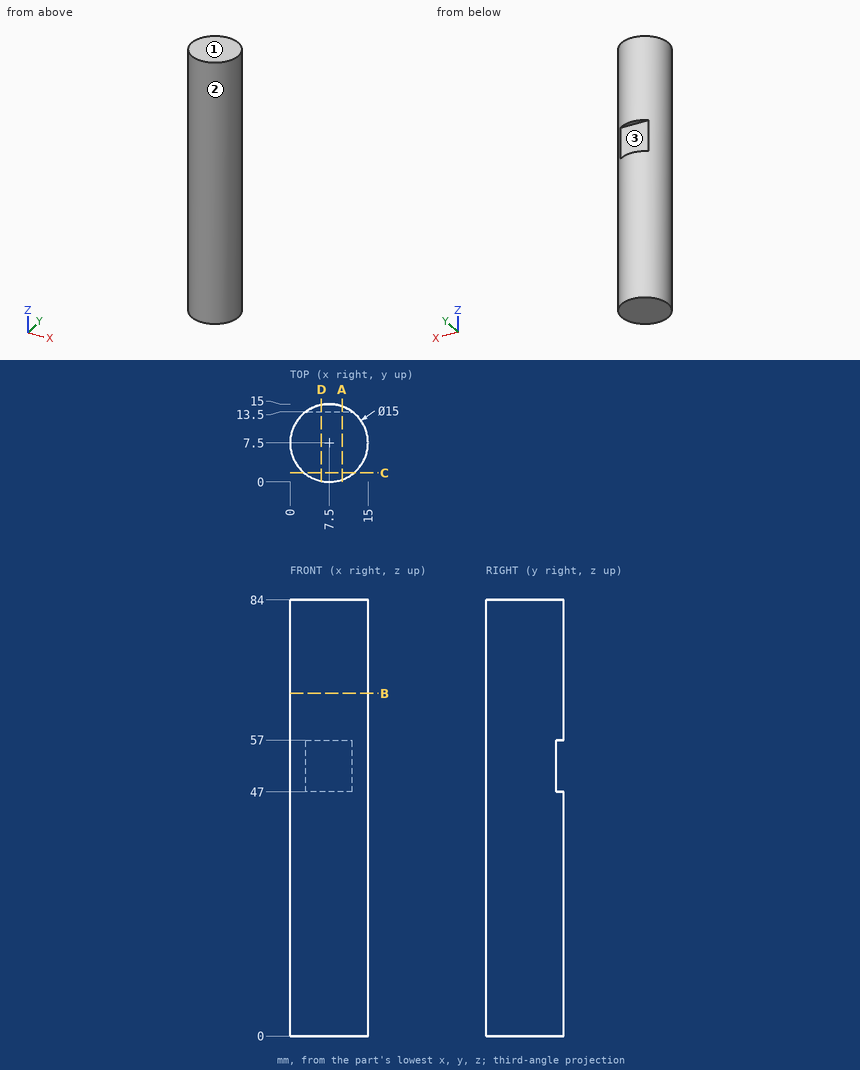
Print and shaded views of the part. All mm, measured from the part's lowest x, y and z. Give positions to 0.01 mm unless a question says otherwise; leave off trailing zeros. Loops run counter-clockwise (first coordinate to the right, second up) from the corner with the lowest first, then second, coordinate; pieces in that order, holes last.
1) Pull direction Z, two halves, no side cores. Call the marked faces 1, 2 and 3: +Z half, -Z half, draft (parallel to the pull), parting line (faces both ways), or undercut.
2) Wall check: line 1 (Z direction, x = 9, y = 13.75); line 2 (Y direction, x = 7, z = 50.5); line 3 (Y direction, x = 7, z = 35.5). Give the ranges that are in metal, low to high.
3) Flat gauge pins, fed straight in: pin 1 Ø3 at (x, z) = (4.5, 27) entering from +Y; pin 2 Ø2 at (y, z) = (10.5, 60.5) entering from -X; pin 3 Ø4.5 at (x, z) = (7.5, 52) entering from +Y. Where does each tip first touch, or does it go through?
4) Saw through at A-A (x = 10). Write the cut outline in (y, z), plus the area to 3 significant figures.
5) Saw through at C-C (y = 1.75). Write the cut outline in (x, z).
6) Saw through at B-B (z = 66). Write the cut outline in (x, y), plus the area to 3 significant figures.
7) Saw through at D-D (x = 6). Write the cut outline in (y, z), plus the area to 3 significant figures.
Answer block:
1. face 1: +Z half
1. face 2: draft
1. face 3: undercut
2. line 1: z = 0 to 47, 57 to 84
2. line 2: y = 0.02 to 13.5
2. line 3: y = 0.02 to 14.98
3. pin 1: stops at y = 14.85
3. pin 2: stops at x = 0.27
3. pin 3: stops at y = 13.5
4. outline: (0.43, 0) - (14.57, 0) - (14.57, 47) - (13.5, 47) - (13.5, 57) - (14.57, 57) - (14.57, 84) - (0.43, 84) - close
4. area: 1,180 mm2
5. outline: (2.68, 0) - (12.32, 0) - (12.32, 84) - (2.68, 84) - close
6. outline: circle Ø15 at (7.5, 7.5)
6. area: 177 mm2
7. outline: (0.15, 0) - (14.85, 0) - (14.85, 47) - (13.5, 47) - (13.5, 57) - (14.85, 57) - (14.85, 84) - (0.15, 84) - close
7. area: 1,220 mm2
